Check sheet for the drawn part. Datum: minimum x, y, z corner. Units: mm. A direction names the side the tool comes from. Coordinates: 2 decimals unless noted, no trailing zeros. Order: outer loops, then holes, each group sorted by start corner. A loop starts at its lowest first (then second) coordinate and runs counter-clockwise, first axis right, second up.
1. Draft check along X on the marked faces 1, 2 and 3. Enter one of: released by +X, released by -X, zero draft, split by the parting line, or undercut.
2. Cross-section at D-D (y = 32.5). Enter the section's corners in (x, z), then the cut area to 3 significant figures.
3. Cross-section at C-C (z = 28). Enter the section's corners in (x, y).
4. Cross-section at B-B (z = 20). Enter the section's corners in (x, y).
5. Thickness scan on line 1 (Y direction, x = 22.25, z = 7); line 2 (X direction, y = 6, z = 4); line 3 (Z direction, x = 13, y = 18.25). Record the ranges inside material, lowest first.
6. Gauge pin test, flat ends, axial feed: pin 1 Ø6 at (x, z) = (14.5, 24) entering from -Y; pin 2 Ø8 at (x, y) = (8.5, 6) entering from -Z; pin 3 Ø9 at (x, y) = (7, 36.5) entering from +Z; pin 4 Ø1.5 at (x, z) = (25.5, 13.5) entering from -Y. Record the tip position at first contact, or that the pin passes through.
7. Set-up check for the marked faces 4, 5, 6, 7 and 8: record each of +Z, -Z, +X, -X, +Y, -Y from which the full face is reachable in a straight line by a thin tool's end or side.
8. Cross-section at A-A (x = 5). Enter the section's corners in (y, z).
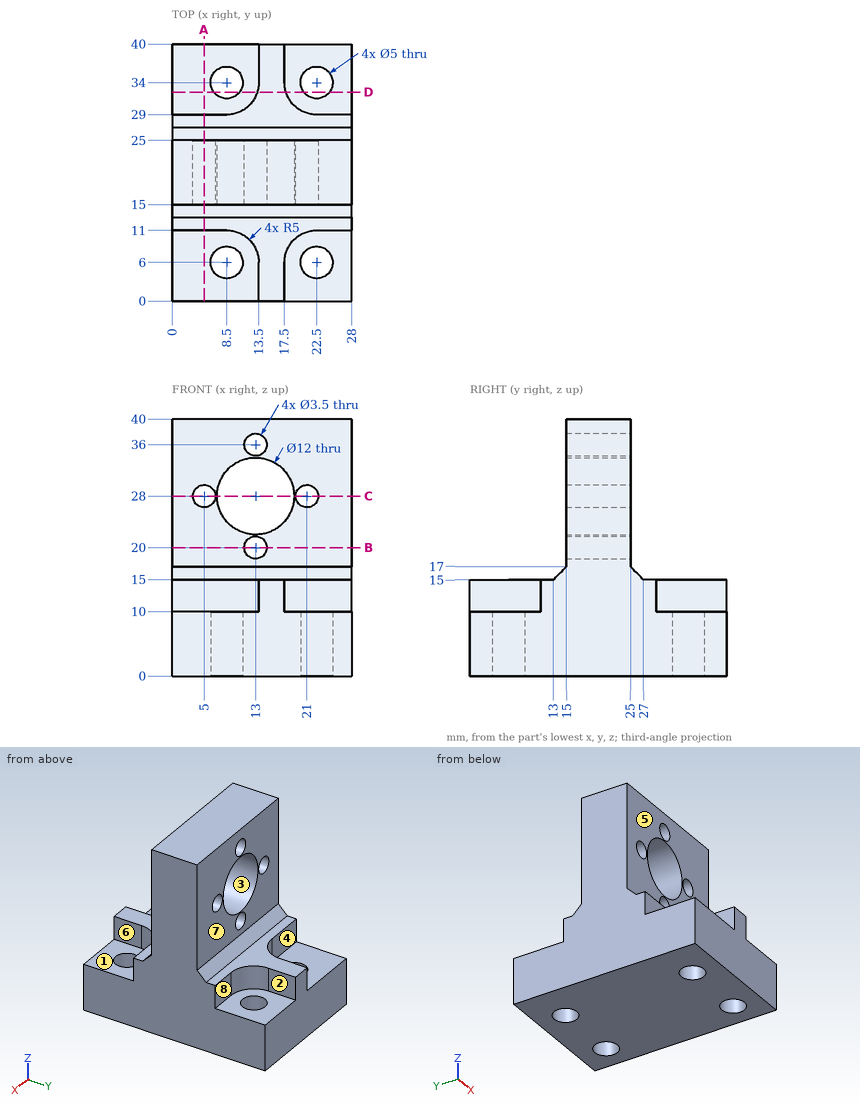
Data:
1. face 1: zero draft
1. face 2: released by +X
1. face 3: undercut
2. outline: (0, 0) - (6.5, 0) - (6.5, 10) - (0, 10) - close; (10.5, 0) - (20.5, 0) - (20.5, 10) - (17.73, 10) - (17.73, 15) - (13.27, 15) - (13.27, 10) - (10.5, 10) - close; (24.5, 0) - (28, 0) - (28, 10) - (24.5, 10) - close
2. area: 222 mm2
3. outline: (0, 15) - (3.25, 15) - (3.25, 25) - (0, 25) - close; (6.75, 15) - (7, 15) - (7, 25) - (6.75, 25) - close; (19, 15) - (19.25, 15) - (19.25, 25) - (19, 25) - close; (22.75, 15) - (28, 15) - (28, 25) - (22.75, 25) - close
4. outline: (0, 15) - (11.25, 15) - (11.25, 25) - (0, 25) - close; (14.75, 15) - (28, 15) - (28, 25) - (14.75, 25) - close
5. line 1: y = 0 to 3.51, 8.49 to 31.51, 36.49 to 40
5. line 2: x = 0 to 6, 11 to 20, 25 to 28
5. line 3: z = 0 to 18.25, 21.75 to 22, 34 to 34.25, 37.75 to 40
6. pin 1: stops at y = 15
6. pin 2: stops at z = 0
6. pin 3: stops at z = 10
6. pin 4: stops at y = 11
7. face 4: +Z, -X, +Y
7. face 5: +Z, +X, -X, -Y
7. face 6: +Z, +X, -Y
7. face 7: +Z, +X, -X, +Y
7. face 8: +Z, +X, +Y
8. outline: (0, 0) - (40, 0) - (40, 10) - (29, 10) - (29, 15) - (27, 15) - (25, 17) - (25, 26.25) - (15, 26.25) - (15, 17) - (13, 15) - (11, 15) - (11, 10) - (0, 10) - close; (15, 29.75) - (25, 29.75) - (25, 40) - (15, 40) - close
